Input: dimensioned drawing with shaded views. Units: mm. Origin: part minimum x, y, z. A direction names the side the tool comes from. Coordinates: 2 decimals unless noted, no trailing zeros. Loops run counter-clockwise (first coordinate to the right, second up) from the corner with the lowest first, then second, coordinate; pieces in that order, holes last.
(1) Contact query for flat-ended pins moving along their axis: P1, Ø4, axis at y = 8, z = 26, coming from the +X side; P2, Ø1.8, axis at y = 5.5, z = 13, coming from the +X side. Output: stop coordinate, or through.
(2) Line query: L1, parallel to Z at x = 29.05, y = 7; L2, parallel to X at y = 2.05, z = 15; L3, parallel to X at y = 7, z = 28.5. Output: solid intervals per line, ascending.
(3) Section C-C, the plane x = 29.05. Return loops of the section in (y, z).
(4) Section B-B, the plane y = 8.75. Return loops of the section in (x, z).
(5) Section D-D, the plane z = 7.5. Return loops of the section in (x, y) (1 decimal), then the cut area to 3 significant figures.
(6) Set-up query: the marked faces 4, 5 and 6. Return all of +Z, -Z, +X, -X, +Y, -Y with unobstructed straight access to the full face (end or side cutting, diameter ignored); none if empty.
(7) Section A-A, the plane z = 15. Return loops of the section in (x, y), then the cut area to 3 significant figures.
(8) Mould query, pull axis Y, two halves, no side actions, for the marked faces 1, 2 and 3. Classes: released by +Y, released by -Y, zero draft, split by the parting line, or undercut.
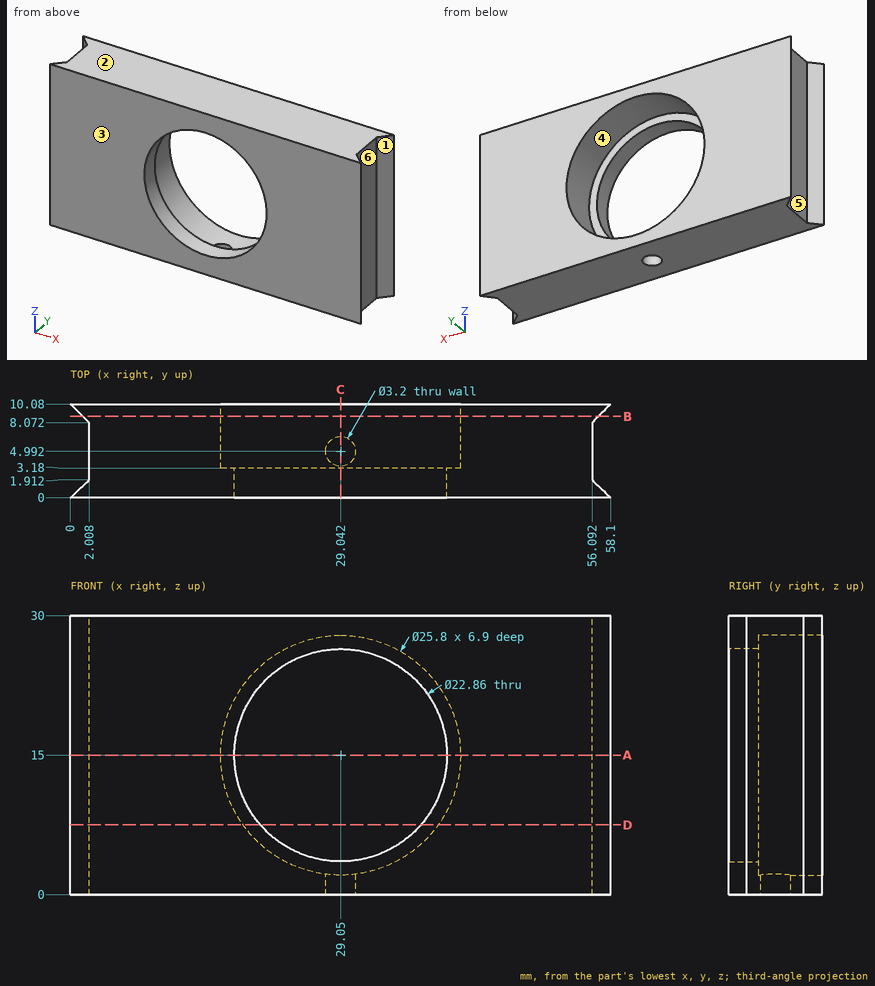
Report:
1. P1: stops at x = 58.02
1. P2: stops at x = 56.09
2. L1: z = 0 to 2.1, 27.9 to 30
2. L2: x = 2.01 to 17.62, 40.48 to 56.09
2. L3: x = 2.01 to 56.09
3. outline: (0, 0) - (3.39, 0) - (3.39, 2.1) - (3.18, 2.1) - (3.18, 3.57) - (0, 3.57) - close; (0, 26.43) - (3.18, 26.43) - (3.18, 27.9) - (10.08, 27.9) - (10.08, 30) - (0, 30) - close; (6.59, 0) - (10.08, 0) - (10.08, 2.1) - (6.59, 2.1) - close
4. outline: (1.33, 0) - (56.77, 0) - (56.77, 30) - (1.33, 30) - close; hole circle Ø25.8 at (29.05, 15)
5. outline: (0, 0) - (20.4, 0) - (20.4, 3.2) - (18.6, 3.2) - (18.6, 10.1) - (0, 10.1) - (2, 8.1) - (2, 1.9) - close; (37.7, 0) - (58.1, 0) - (56.1, 1.9) - (56.1, 8.1) - (58.1, 10.1) - (39.5, 10.1) - (39.5, 3.2) - (37.7, 3.2) - close
5. area: 353 mm2
6. face 4: +Y
6. face 5: +Z, -Z, -X
6. face 6: +Z, -Z, +X
7. outline: (0, 0) - (17.62, 0) - (17.62, 3.18) - (16.15, 3.18) - (16.15, 10.08) - (0, 10.08) - (2.01, 8.07) - (2.01, 1.91) - close; (40.48, 0) - (58.1, 0) - (56.09, 1.91) - (56.09, 8.07) - (58.1, 10.08) - (41.95, 10.08) - (41.95, 3.18) - (40.48, 3.18) - close
7. area: 302 mm2
8. face 1: undercut
8. face 2: zero draft
8. face 3: released by -Y
